from build123d import *

# Parameters (mm, degrees)
BOSS_EXTRUDE1_DEPTH = 32
SKETCH2_W           = 32
SKETCH2_H           = 297.871609812
BOSS_EXTRUDE2_DEPTH = 4
SKETCH3_W           = 32
SKETCH3_H           = 297.871609812
BOSS_EXTRUDE3_DEPTH = 4


with BuildPart() as part:
    # Sketch1 → Boss-Extrude1 (new body)
    with BuildSketch(Plane.XY):
        with BuildLine():
            Line((-78.105635002, -6.676845901), (-52.734667386, -303.466013381))
            ThreePointArc((-52.734667386, -303.466013381), (0, -351.885), (52.734667386, -303.466013381))
            Line((52.734667386, -303.466013381), (78.105635002, -6.676845901))
            ThreePointArc((78.105635002, -6.676845901), (0, 78.3905), (-78.105635002, -6.676845901))
        make_face()
        with BuildLine():
            Line((-76.112902847, -6.506497557), (-50.741935231, -303.295665038))
            ThreePointArc((-50.741935231, -303.295665038), (0, -349.885), (50.741935231, -303.295665038))
            Line((50.741935231, -303.295665038), (76.112902847, -6.506497557))
            ThreePointArc((76.112902847, -6.506497557), (0, 76.3905), (-76.112902847, -6.506497557))
        make_face(mode=Mode.SUBTRACT)
    extrude(amount=BOSS_EXTRUDE1_DEPTH)

    # Sketch2 → Boss-Extrude2 (add)
    with BuildSketch(Plane(origin=(76.112902847, -6.506497557, 0), x_dir=(0, 0, 1), z_dir=(-0.996366077547994, 0.08517417162276966, 0))):
        with Locations((16, -148.935804906)):
            Rectangle(SKETCH2_W, SKETCH2_H)
    extrude(amount=BOSS_EXTRUDE2_DEPTH)

    # Sketch3 → Boss-Extrude3 (add)
    with BuildSketch(Plane(origin=(-76.112902847, -6.506497557, 0), x_dir=(0, 0, -1), z_dir=(0.9963660775479939, 0.08517417162276988, 0))):
        with Locations((-16, -148.935804906)):
            Rectangle(SKETCH3_W, SKETCH3_H)
    extrude(amount=BOSS_EXTRUDE3_DEPTH)


solid = part.part
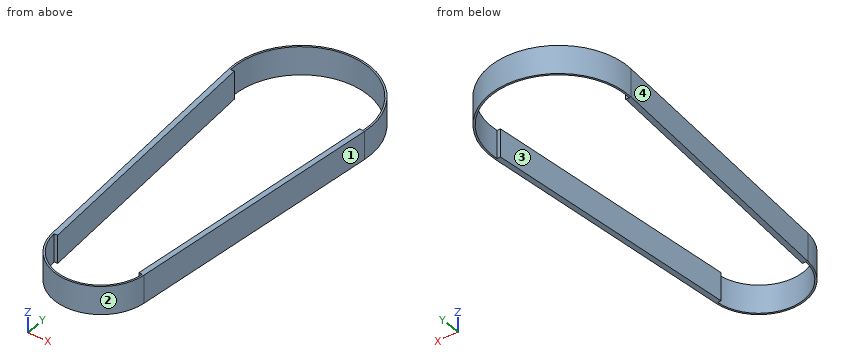
Input: part model. Units: mm. Frame: model coordinates. Face numbers are marked on the shaded views. Give positions to 0.01 mm unless a question says otherwise; leave off trailing zeros. Loops run counter-clockwise (first coordinate to the right, second up) from the corner with the lowest first, then second, coordinate; pieces in that order, holes last. Notation, with made-up numbers: (89.5, 6.25) - (107.5, 6.25) arc R6 cw to (107.5, 10.25) - close; hole circle Ø10 at (72, -13). An arc over 180 degrees is marked (long way). Use CSV: the item, a comma, the result in double quotes. Start each with the question number.
Item 1: Section B-B on z = 25. Return loops of the section in (x, y), then the cut area to 3 significant figures.
Item 2: Section A-A on x = 0. Return loops of the section in (y, z) (1 decimal), then the cut area to 3 significant figures.
Item 3: Line query: line 1 (X direction, y = 0, z = 18.5); line 2 (Y direction, x = -16.5, z = 18.5); line 3 (X direction, y = -228, z = 12). Output: solid intervals per line, ascending.
Item 4: Contact query for flat-ended pins moving along their axis: P1, Ø10, axis at y = -54, z = 4.5, coming from the +X side; P2, Ø10, axis at x = 52.5, z = 9.5, coming from the -Y side; P3, Ø4, axis at y = -217.5, z = 16, coming from the +X side. Output: stop coordinate, or through.
Item 5: Mould query, pull axis X, two halves, no side actions, for the marked faces 1, 2, 3 and 4. Classes: pulls with the +X half, pulls with the -X half, needs draft (parallel to the pull), parting line crosses it, or undercut.
Item 6: Section C-C on y = 0. Return loops of the section in (x, z).
Ans:
1,outline,"(-78.11, -6.68) - (-52.73, -303.47) arc R52.93 ccw to (52.73, -303.47) - (78.11, -6.68) arc R78.39 ccw (long way) to start; hole (-76.11, -6.51) - (-72.13, -6.17) - (-46.76, -302.95) - (-50.74, -303.3) arc R50.93 ccw to (50.74, -303.3) - (46.76, -302.95) - (72.13, -6.17) - (76.11, -6.51) arc R76.39 ccw (long way) to start"
1,area,"4,400 mm2"
2,outline,"(-351.9, 0) - (-349.9, 0) - (-349.9, 32) - (-351.9, 32) - close; (76.4, 0) - (78.4, 0) - (78.4, 32) - (76.4, 32) - close"
2,area,"128 mm2"
3,line 1,"x = -78.39 to -76.39, 76.39 to 78.39"
3,line 2,"y = -349.25 to -347.14, 74.59 to 76.63"
3,line 3,"x = -59.19 to -53.16, 53.16 to 59.19"
4,P1,"stops at x = 74.49"
4,P2,"stops at y = -322.3"
4,P3,"stops at x = 60.25"
5,face 1,"pulls with the +X half"
5,face 2,"parting line crosses it"
5,face 3,"undercut"
5,face 4,"pulls with the -X half"
6,outline,"(-78.39, 0) - (-76.39, 0) - (-76.39, 32) - (-78.39, 32) - close; (76.39, 0) - (78.39, 0) - (78.39, 32) - (76.39, 32) - close"
